Can you work these out from the model? Positions are in its coordinate system, mm. Give positions to 0.01 mm unless a question says otherwise; leave off trailing zeros. Order: outer loops, then holes, each group sorted by start corner. A loop starts at its lowest first (then second) coordinate and runs counter-clockwise, first axis right, second up. Notation, with made-up numbers: M 38,-39 L 78,-39 A13 cw 78,-20 Z; hole C 2,70.5 d6. An arc over 180 degrees is marked long. Write each question's results on one line, items separated by ' | '.
Autodesk Inventor part; units mm, degrees
ref_plane "YZ Plane" through (0, 0, 0) normal (1, 0, 0) x (0, 1, 0)
ref_plane "XZ Plane" through (0, 0, 0) normal (0, 1, 0) x (-1, 0, 0)
ref_plane "XY Plane" through (0, 0, 0) normal (0, 0, 1) x (1, 0, 0)
sketch "Esboço1" plane through (0, 0, 0) normal (0, 1, 0) x (-1, 0, 0)
  line L0 (0, 0) -> (300, 0)
  line L1 (300, 0) -> (300, -320)
  line L2 (300, -320) -> (0, -320)
  line L3 (0, -320) -> (0, 0)
  dimension "d0" = 300
  dimension "d1" = 320
extrude "Extrusão1" add sketch "Esboço1" along normal blind 10
sketch "Sketch2" plane through (0, 10, 0) normal (0, 1, 0) x (1, 0, 0)
  line L0 (-300, 320) -> (-300, 0)
  line L1 (-300, 0) -> (0, 0)
  line L2 (0, 320) -> (-300, 320)
  line L3 (0, 0) -> (0, 320)
  point P0 (-182, 239.6)
  point P1 (-182, 303.6)
  point P2 (-118, 239.6)
  point P3 (-118, 303.6)
  point P4 (-211, 281.6)
  point P5 (-89, 281.6)
  point P6 (-211, 261.6)
  point P7 (-89, 261.6)
  point P8 (-240, 28.1)
  point P9 (-240, 208.1)
  point P10 (-60, 28.1)
  point P11 (-60, 208.1)
  dimension "d16" = 64
  dimension "d17" = 64
  dimension "d18" = 300
  dimension "d19" = 320
  dimension "d20" = 16.4
  dimension "d21" = 118
  dimension "d22" = 122
  dimension "d23" = 20
  dimension "d24" = 38.4
  dimension "d25" = 89
  dimension "d26" = 180
  dimension "d27" = 180
  dimension "d28" = 60
  dimension "d29" = 28.1
hole "Hole1" at (-60, 10, -208.1) at (-60, 10, -28.1) at (-240, 10, -208.1) at (-240, 10, -28.1) at (-89, 10, -261.6) at (-211, 10, -261.6) at (-89, 10, -281.6) at (-211, 10, -281.6) at (-118, 10, -303.6) at (-118, 10, -239.6) at (-182, 10, -303.6) at (-182, 10, -239.6) direction (0, -1, 0) diameter 5 end through all
sketch "Sketch3" plane through (0, 10, 0) normal (0, 1, 0) x (1, 0, 0)
  line L0 (-300, 320) -> (-300, 0)
  line L1 (-300, 0) -> (0, 0)
  point P0 (-280, 20)
  point P1 (-280, 300)
  point P2 (-20, 20)
  point P3 (-20, 300)
  dimension "d41" = 280
  dimension "d42" = 260
  dimension "d43" = 320
  dimension "d44" = 300
  dimension "d45" = 20
  dimension "d46" = 20
hole "Hole2" at (-20, 10, -300) at (-20, 10, -20) at (-280, 10, -300) at (-280, 10, -20) direction (0, -1, 0) diameter 7.134 end through all
equation "\"d35\" = Espessura"
equation "\"Raio_vergadura\" = Espessura"
equation "\"Largura_alívio_de_vergadura\" = Espessura"
equation "\"Profundidade_alívio_de_vergadura\" = 0.5 * Espessura"
equation "\"Tamanho_alívio_de_dobra\" = 4 * Espessura"
equation "\"Remanescente_mínimo\" = 2 * Espessura"
equation "\"Raiodetransição\" = Raio_vergadura"
equation "\"Tamanho_de_raio_de_Jacobi\" = Raio_vergadura"
equation "\"TamanhoFolga\" = Espessura"
properties part number "Base madeira" material "Wood (Oak)"
(1) We'd pull the mould along Z, two halves only. Please class faces 1 (the face through (-18.634, 4.93, -296.705)), 2 (the face through (-148, 5, 0)), 3 (the face through (-300, 5, -158)): +Z half, -Z half, draft (parallel to the pull), parting line (faces both ways), or undercut.
Data:
face 1: undercut | face 2: +Z half | face 3: draft
(2) Imagine slicing it at A-A, the plane x = -20. Write out the boundary of the cut face in (y, z), plus the area to 3 significant figures.
Data:
outline: M 0,-320 L 10,-320 L 10,-303.57 L 0,-303.57 Z; M 0,-296.43 L 10,-296.43 L 10,-23.57 L 0,-23.57 Z; M 0,-16.43 L 10,-16.43 L 10,0 L 0,0 Z | area: 3,060 mm2
(3) I need wall thicknesses on L1, parallel to X at y = 3.25, z = -28.1; L2, parallel to Z at x = -60, y = 6.5; L3, parallel to X at y = 6.75, z = -303.6. Which ranges of each line are inside material? Lowest first, please. Write a range as from..to.
Data:
L1: x = -300..-242.5, -237.5..-62.5, -57.5..0 | L2: z = -320..-210.6, -205.6..-30.6, -25.6..0 | L3: x = -300..-184.5, -179.5..-120.5, -115.5..0
